The drawing under review shows one solid part. Ordinate dimensions are in mm from its lowest x, y, z. A direction names the side the tool comes from. Round coordinates to 2 decimals unless told otherwise and drop trailing zeros. Write each loop counter-clockwise with the first axis right and the second up, starting at its lowest first coordinate (ties: lowest second). Pieces come first, ordered by that corner, then holes.
Item 1: Add section B-B (y = 1.5). Give the boundary of the cut face in (x, z), plus the area to 3 significant figures.
Item 2: Add section C-C (z = 6.15). Give the boundary of the cut face in (x, y), plus the area to 3 significant figures.
Item 3: Draft analysis for pull direction X (two halves, no side actions). For the marked faces 1, 2 and 3, state which applies: +X half, -X half, draft (parallel to the pull), parting line (faces both ways), or undercut.
Item 4: Add section A-A (x = 38.5). Give the boundary of the cut face in (y, z).
Item 5: Machinability: for the marked faces 4, 5 and 6, which of the approach directions +Z, -Z, +X, -X, +Y, -Y give a long, thin tool a straight path to every point of the face, cutting with its end or side? Answer none if there is none.
Item 6: To check wall thickness, follow L1, parallel to Z at x = 13, y = 6.5; L2, parallel to X at y = 1.5, z = 8; L3, parallel to X at y = 0.5, z = 19. State the ranges of each line that lie inside material, in increasing order.
Item 7: Add section D-D (x = 18). Give the boundary of the cut face in (y, z), plus the area to 3 significant figures.
Item 8: Clearance check with flat-ended pins moving along their axes: pin 1 Ø3 at (y, z) = (6, 13.5) entering from +X; pin 2 Ø2 at (x, y) = (32, 5) entering from -Z. State where each tip first meets the part, or that it passes through.
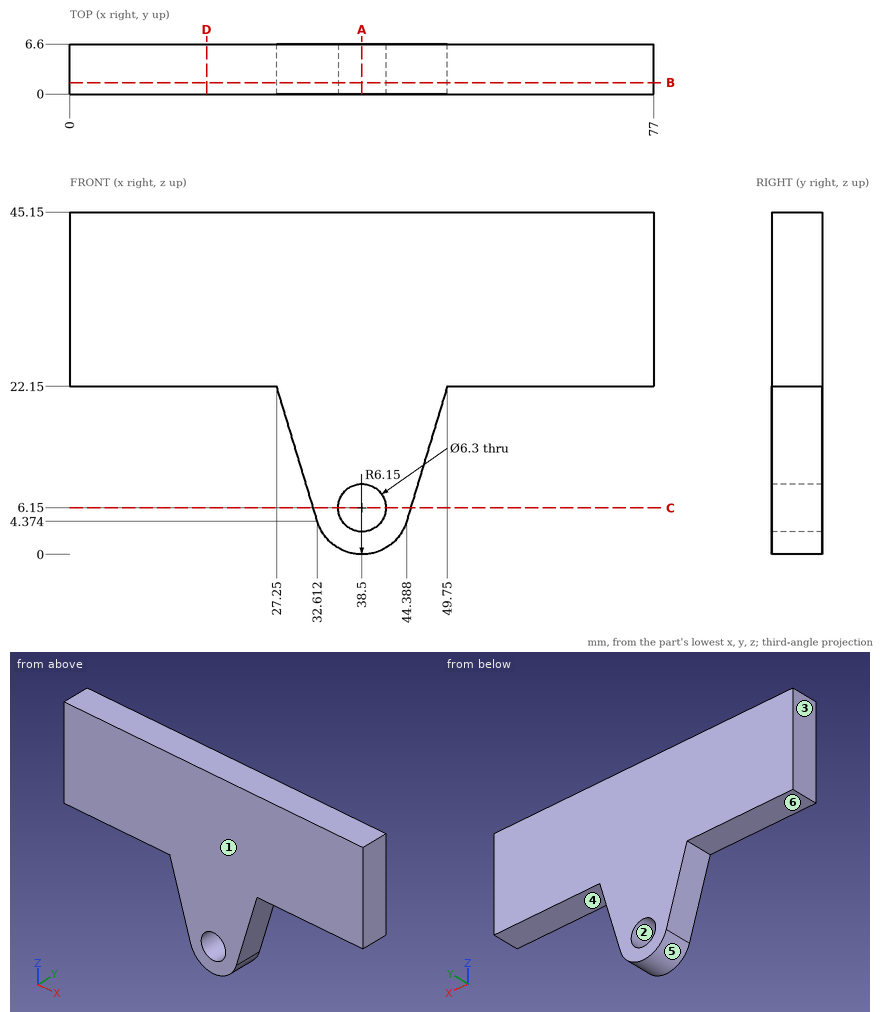
Numbers:
1. outline: (0, 22.15) - (27.25, 22.15) - (32.61, 4.37) arc R6.15 ccw to (44.39, 4.37) - (49.75, 22.15) - (77, 22.15) - (77, 45.15) - (0, 45.15) - close; hole circle Ø6.3 at (38.5, 6.15)
1. area: 2,080 mm2
2. outline: (32.08, 0) - (35.35, 0) - (35.35, 6.6) - (32.08, 6.6) - close; (41.65, 0) - (44.92, 0) - (44.92, 6.6) - (41.65, 6.6) - close
2. area: 43.2 mm2
3. face 1: draft
3. face 2: undercut
3. face 3: -X half
4. outline: (0, 0) - (6.6, 0) - (6.6, 3) - (0, 3) - close; (0, 9.3) - (6.6, 9.3) - (6.6, 45.15) - (0, 45.15) - close
5. face 4: -Z, +X, +Y, -Y
5. face 5: -Z, +Y, -Y
5. face 6: -Z, -X, +Y, -Y
6. L1: z = 22.15 to 45.15
6. L2: x = 31.52 to 35.95, 41.05 to 45.48
6. L3: x = 28.2 to 48.8
7. outline: (0, 22.15) - (6.6, 22.15) - (6.6, 45.15) - (0, 45.15) - close
7. area: 152 mm2
8. pin 1: stops at x = 47.59
8. pin 2: stops at z = 3.4
